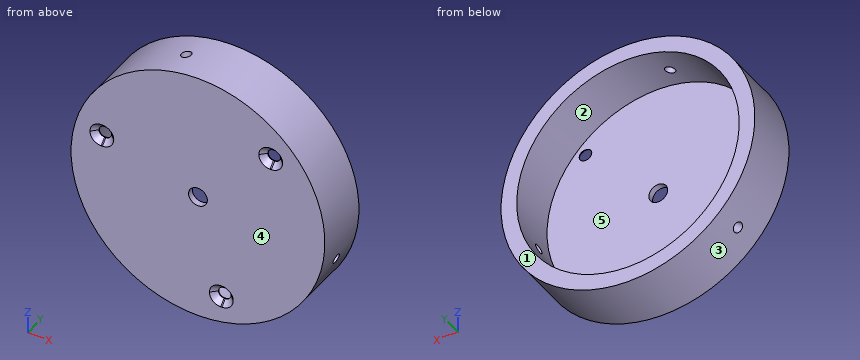
```python
from build123d import *

# Parameters (mm, degrees)
SKETCH1_R                                     = 20.25
BOSS_EXTRUDE1_DEPTH                           = 9
SKETCH2_R                                     = 17.75
CUT_EXTRUDE1_DEPTH                            = 8
CSK_START                                     = -1
CSK_SLOT_FOR_M1_6_COUNTERSUNK_FLAT_HEAD_DEPTH = 3
CIRPATTERN1_START                             = -1
CIRPATTERN1_DEPTH                             = 3
SKETCH5_R                                     = 1.5
CUT_EXTRUDE2_DEPTH                            = 8
CIRPATTERN2_COUNT                             = 3


with BuildPart() as part:
    # Sketch1 → Boss-Extrude1 (new body)
    with BuildSketch(Plane(origin=(0, 0, 0), x_dir=(1, 0, 0), z_dir=(0, 1, 0))):
        with Locations(Location((0, 0, 0), (0, 0, 270))):
            Circle(SKETCH1_R)
    extrude(amount=BOSS_EXTRUDE1_DEPTH)

    # Sketch2 → Cut-Extrude1 (cut)
    with BuildSketch(Plane(origin=(0, 9, 0), x_dir=(1, 0, 0), z_dir=(0, 1, 0))):
        with Locations(Location((0, 0, 0), (0, 0, 270))):
            Circle(SKETCH2_R)
    extrude(amount=-CUT_EXTRUDE1_DEPTH, mode=Mode.SUBTRACT)

    # CSK SLOT for M1.6 Countersunk Flat Head: read off the stored shape, not the designer's step
    # CSK SLOT for M1.6 Countersunk Flat H 2 → CSK SLOT for M1.6 Countersunk Flat Head (cut)
    with BuildSketch(Plane(origin=(0, 0, 0), x_dir=(1, 0, 0), z_dir=(0, 1, 0)).offset(CSK_START)):
        with BuildLine():
            ThreePointArc((11.709715894, -11.90974554), (12.609715894, -11.00974554), (11.709715894, -10.10974554))
            Line((11.709715894, -10.10974554), (11.509715894, -10.10974554))
            ThreePointArc((11.509715894, -10.10974554), (10.609715894, -11.00974554), (11.509715894, -11.90974554))
            Line((11.509715894, -11.90974554), (11.709715894, -11.90974554))
        make_face()
    extrude(amount=CSK_SLOT_FOR_M1_6_COUNTERSUNK_FLAT_HEAD_DEPTH, mode=Mode.SUBTRACT)

    # CSK SLOT for M1.6 Countersunk Flat H 3: loft between two sections, ruled curve by curve
    csk_slot_for_m1_6_countersunk_flat_h_3_from = [
        Edge.make_three_point_arc((11.709715894, 0.9, 10.10974554), (12.346111997, 0.9, 10.373349437), (12.609715894, 0.9, 11.00974554)),
        Edge.make_three_point_arc((12.609715894, 0.9, 11.00974554), (12.346111997, 0.9, 11.646141643), (11.709715894, 0.9, 11.90974554)),
        Edge.make_three_point_arc((11.509715894, 0.9, 11.90974554), (10.873319791, 0.9, 11.646141643), (10.609715894, 0.9, 11.00974554)),
        Edge.make_three_point_arc((10.609715894, 0.9, 11.00974554), (10.873319791, 0.9, 10.373349437), (11.509715894, 0.9, 10.10974554)),
        Edge.make_line((11.709715894, 0.9, 11.90974554), (11.509715894, 0.9, 11.90974554)),
        Edge.make_line((11.709715894, 0.9, 10.10974554), (11.509715894, 0.9, 10.10974554)),
    ]
    csk_slot_for_m1_6_countersunk_flat_h_3_to = [
        Edge.make_three_point_arc((11.709715894, 0, 9.20974554), (12.9825081, 0, 9.736953334), (13.509715894, 0, 11.00974554)),
        Edge.make_three_point_arc((13.509715894, 0, 11.00974554), (12.9825081, 0, 12.282537747), (11.709715894, 0, 12.80974554)),
        Edge.make_three_point_arc((11.509715894, 0, 12.80974554), (10.236923688, 0, 12.282537747), (9.709715894, 0, 11.00974554)),
        Edge.make_three_point_arc((9.709715894, 0, 11.00974554), (10.236923688, 0, 9.736953334), (11.509715894, 0, 9.20974554)),
        Edge.make_line((11.709715894, 0, 12.80974554), (11.509715894, 0, 12.80974554)),
        Edge.make_line((11.709715894, 0, 9.20974554), (11.509715894, 0, 9.20974554)),
    ]
    csk_slot_for_m1_6_countersunk_flat_h_3 = Solid(Shell([*[Face.make_surface_from_curves(csk_slot_for_m1_6_countersunk_flat_h_3_from[k], csk_slot_for_m1_6_countersunk_flat_h_3_to[k]) for k in range(6)], Face(Wire(csk_slot_for_m1_6_countersunk_flat_h_3_from)), Face(Wire(csk_slot_for_m1_6_countersunk_flat_h_3_to))]))
    add(csk_slot_for_m1_6_countersunk_flat_h_3, mode=Mode.SUBTRACT)

    # CirPattern1: read off the stored shape, not the designer's step
    # CirPattern1 outline → CirPattern1 (cut)
    with BuildSketch(Plane(origin=(0, 0, 0), x_dir=(1, 0, 0), z_dir=(0, 1, 0)).offset(CIRPATTERN1_START)):
        with BuildLine():
            ThreePointArc((-15.239577274, -5.449436125), (-14.339577274, -4.549436125), (-15.239577274, -3.649436125))
            Line((-15.239577274, -3.649436125), (-15.439577274, -3.649436125))
            ThreePointArc((-15.439577274, -3.649436125), (-16.339577274, -4.549436125), (-15.439577274, -5.449436125))
            Line((-15.439577274, -5.449436125), (-15.239577274, -5.449436125))
        make_face()
        with BuildLine():
            ThreePointArc((3.82986138, 14.659181665), (4.72986138, 15.559181665), (3.82986138, 16.459181665))
            Line((3.82986138, 16.459181665), (3.62986138, 16.459181665))
            ThreePointArc((3.62986138, 16.459181665), (2.72986138, 15.559181665), (3.62986138, 14.659181665))
            Line((3.62986138, 14.659181665), (3.82986138, 14.659181665))
        make_face()
    extrude(amount=CIRPATTERN1_DEPTH, mode=Mode.SUBTRACT)

    # CirPattern1 2: loft between two sections, ruled curve by curve
    cirpattern1_2_from = [
        Edge.make_three_point_arc((-15.239577274, 0.9, 3.649436125), (-14.603181171, 0.9, 3.913040022), (-14.339577274, 0.9, 4.549436125)),
        Edge.make_three_point_arc((-14.339577274, 0.9, 4.549436125), (-14.603181171, 0.9, 5.185832228), (-15.239577274, 0.9, 5.449436125)),
        Edge.make_three_point_arc((-15.439577274, 0.9, 5.449436125), (-16.075973377, 0.9, 5.185832228), (-16.339577274, 0.9, 4.549436125)),
        Edge.make_three_point_arc((-16.339577274, 0.9, 4.549436125), (-16.075973377, 0.9, 3.913040022), (-15.439577274, 0.9, 3.649436125)),
        Edge.make_line((-15.239577274, 0.9, 5.449436125), (-15.439577274, 0.9, 5.449436125)),
        Edge.make_line((-15.239577274, 0.9, 3.649436125), (-15.439577274, 0.9, 3.649436125)),
    ]
    cirpattern1_2_to = [
        Edge.make_three_point_arc((-15.239577274, 0, 2.749436125), (-13.966785068, 0, 3.276643918), (-13.439577274, 0, 4.549436125)),
        Edge.make_three_point_arc((-13.439577274, 0, 4.549436125), (-13.966785068, 0, 5.822228331), (-15.239577274, 0, 6.349436125)),
        Edge.make_three_point_arc((-15.439577274, 0, 6.349436125), (-16.71236948, 0, 5.822228331), (-17.239577274, 0, 4.549436125)),
        Edge.make_three_point_arc((-17.239577274, 0, 4.549436125), (-16.71236948, 0, 3.276643918), (-15.439577274, 0, 2.749436125)),
        Edge.make_line((-15.239577274, 0, 6.349436125), (-15.439577274, 0, 6.349436125)),
        Edge.make_line((-15.239577274, 0, 2.749436125), (-15.439577274, 0, 2.749436125)),
    ]
    cirpattern1_2 = Solid(Shell([*[Face.make_surface_from_curves(cirpattern1_2_from[k], cirpattern1_2_to[k]) for k in range(6)], Face(Wire(cirpattern1_2_from)), Face(Wire(cirpattern1_2_to))]))
    add(cirpattern1_2, mode=Mode.SUBTRACT)

    # CirPattern1 3: loft between two sections, ruled curve by curve
    cirpattern1_3_from = [
        Edge.make_three_point_arc((3.82986138, 0.9, -16.459181665), (4.466257483, 0.9, -16.195577768), (4.72986138, 0.9, -15.559181665)),
        Edge.make_three_point_arc((4.72986138, 0.9, -15.559181665), (4.466257483, 0.9, -14.922785562), (3.82986138, 0.9, -14.659181665)),
        Edge.make_three_point_arc((3.62986138, 0.9, -14.659181665), (2.993465277, 0.9, -14.922785562), (2.72986138, 0.9, -15.559181665)),
        Edge.make_three_point_arc((2.72986138, 0.9, -15.559181665), (2.993465277, 0.9, -16.195577768), (3.62986138, 0.9, -16.459181665)),
        Edge.make_line((3.82986138, 0.9, -14.659181665), (3.62986138, 0.9, -14.659181665)),
        Edge.make_line((3.82986138, 0.9, -16.459181665), (3.62986138, 0.9, -16.459181665)),
    ]
    cirpattern1_3_to = [
        Edge.make_three_point_arc((3.82986138, 0, -17.359181665), (5.102653586, 0, -16.831973871), (5.62986138, 0, -15.559181665)),
        Edge.make_three_point_arc((5.62986138, 0, -15.559181665), (5.102653586, 0, -14.286389459), (3.82986138, 0, -13.759181665)),
        Edge.make_three_point_arc((3.62986138, 0, -13.759181665), (2.357069174, 0, -14.286389459), (1.82986138, 0, -15.559181665)),
        Edge.make_three_point_arc((1.82986138, 0, -15.559181665), (2.357069174, 0, -16.831973871), (3.62986138, 0, -17.359181665)),
        Edge.make_line((3.82986138, 0, -13.759181665), (3.62986138, 0, -13.759181665)),
        Edge.make_line((3.82986138, 0, -17.359181665), (3.62986138, 0, -17.359181665)),
    ]
    cirpattern1_3 = Solid(Shell([*[Face.make_surface_from_curves(cirpattern1_3_from[k], cirpattern1_3_to[k]) for k in range(6)], Face(Wire(cirpattern1_3_from)), Face(Wire(cirpattern1_3_to))]))
    add(cirpattern1_3, mode=Mode.SUBTRACT)

    # Sketch5 → Cut-Extrude2 (cut)
    with BuildSketch(Plane.XZ):
        with Locations(Location((0, 0, 0), (0, 0, 270))):
            Circle(SKETCH5_R)
    extrude(amount=-CUT_EXTRUDE2_DEPTH, mode=Mode.SUBTRACT)

    # Sketch6 → M2 Tapped Hole1 (revolve, cut)
    with BuildSketch(Plane(origin=(-4.560794248, 4.445790719, 19.729715047), x_dir=(0.974306915892993, 0, 0.22522440729877435), z_dir=(0, 1, 0))):
        Polygon((0, 0), (0, 4.980688495), (0.8, 4.5), (0.8, 0), align=None)
    m2_tapped_hole1 = revolve(axis=Axis((-5.990969234, 4.445790719, 25.916563963), (0.22522440729877433, 0, -0.9743069158929931)), mode=Mode.SUBTRACT)

    # CirPattern2: M2 Tapped Hole1 ×3 about axis
    cirpattern2_axis = Axis((0, 9, 0), (0, -1, 0))
    for i in range(1, CIRPATTERN2_COUNT):
        add(m2_tapped_hole1.rotate(cirpattern2_axis, i * 360 / CIRPATTERN2_COUNT), mode=Mode.SUBTRACT)


solid = part.part
```
CAD build for the part. Positions are in the model's coordinates, mm. Face numbers are marked on the shaded views. A direction names the side the tool comes from. Give positions to 0.01 mm unless a question says otherwise; leave off trailing zeros. Write each loop counter-clockwise with the first axis right and the second up, starting at its lowest first coordinate (ties: lowest second). Pieces come first, ordered by that corner, then holes. Notation, with made-up numbers: (-23, 30) -> (24, 30) arc R28 cw to (24, 50) -> close; hole circle Ø3 at (51.25, 49). An arc over 180 degrees is marked (long way). Write each question's results on one line, items separated by ' | '.
1. Drop flat-ended pins along their axis: P1, Ø5, axis at x = 9, z = -5.5, coming from the +Y side; P2, Ø2, axis at x = -11, y = 4, coming from the -Z side; P3, Ø2.5, axis at x = 0, z = 0, coming from the -Y side; P4, Ø5, axis at y = 8, z = 5, coming from the -X side. Give the stop position or say it passes through.
Geometry check:
P1: y = 1 | P2: z = -17.61 | P3: through | P4: x = -20.1
2. Which spindle directions (+Z, -Z, +X, -X, +Y, -Y) get a long thin tool onto all of the face, cutting with end or side? Do the marked faces 1 and 2. Say none if no direction does.
Geometry check:
face 1: +Z, -Z, +X, -X, +Y | face 2: +Y
3. Cut at C-C, the plane y = 1.5. Write the cut outline in (x, z), then the cut area to 3 significant figures.
Geometry check:
outline: circle Ø40.5 at (0, 0); hole circle Ø35.5 at (0, 0) | area: 298 mm²
4. Cut at A-A, the plane z = 0. Write the cut outline in (x, y), then the cut area to 3 significant figures.
Geometry check:
outline: (-20.25, 0) -> (-1.5, 0) -> (-1.5, 1) -> (-17.75, 1) -> (-17.75, 9) -> (-20.25, 9) -> close; (1.5, 0) -> (20.25, 0) -> (20.25, 9) -> (17.75, 9) -> (17.75, 1) -> (1.5, 1) -> close | area: 77.5 mm²
5. Two-plate mould, pull along Z, no slides. Class the marked faces 3, 4 and 5: pulls with the +Z half, pulls with the -Z half, needs draft (parallel to the pull), parting line crosses it, or undercut.
Geometry check:
face 3: parting line crosses it | face 4: needs draft | face 5: undercut
6. Wall check: probe 1 along X at (y, z) = (3.25, 0); probe 2 along X at (y, z) = (0.75, 0); probe 3 along Y at (x, z) = (-16, -1.5). Give the ranges that are in metal, low to high. Write a range as [from, to].
Geometry check:
probe 1: [-20.25, -17.75], [17.75, 20.25] | probe 2: [-20.25, -1.5], [1.5, 20.25] | probe 3: [0, 1]
7. Cut at B-B, the plane x = 0. Write the cut outline in (y, z), then the cut area to 3 significant figures.
Geometry check:
outline: (0, -20.25) -> (9, -20.25) -> (9, -17.75) -> (1, -17.75) -> (1, -1.5) -> (0, -1.5) -> close; (0, 1.5) -> (1, 1.5) -> (1, 17.75) -> (9, 17.75) -> (9, 20.25) -> (0, 20.25) -> close | area: 77.5 mm²
8. Cut at D-D, the plane x = 7. Write the cut outline in (y, z), then the cut area to 3 significant figures.
Geometry check:
outline: (0, -19) -> (9, -19) -> (9, -16.31) -> (1, -16.31) -> (1, 16.31) -> (9, 16.31) -> (9, 19) -> (0, 19) -> close | area: 81.0 mm²
